Verification items for this drawing (mm, ordinates from the low corner). Coordinates: 2 decimals unless noted, no trailing zeros. Order: outer loops, then holes, each group sorted by start corner. A loop starts at its lowest first (then second) coordinate and runs counter-clockwise, first axis right, second up. Notation, with made-up numbers: (-11, 76.5) - (22, 76.5) arc R30 cw to (22, 106.5) - close; hole circle Ø4 at (34.25, -16.5). An arc over 180 degrees is marked (long way). Use CSV: the item, a comma, the result in double quotes. Start each with the question number.
1) Depth check by flat-ended pin: P1, Ø7.5, axis at x = 17.78, y = 17.78, coming from the +Z side. Enter the tip coordinate at first touch or a pass-through.
2) Sectioned sample at B-B, the plane x = 287.02. Record the cut outline in (y, z).
3) Sectioned sample at A-A, the plane y = 134.62. Record the cut outline in (x, z).
4) Thickness scan on probe 1 along Y at (x, z) = (287.02, 8); probe 2 along Y at (x, z) = (284.5, 10). Record the ranges inside material, lowest first. Write a range as [from, to].
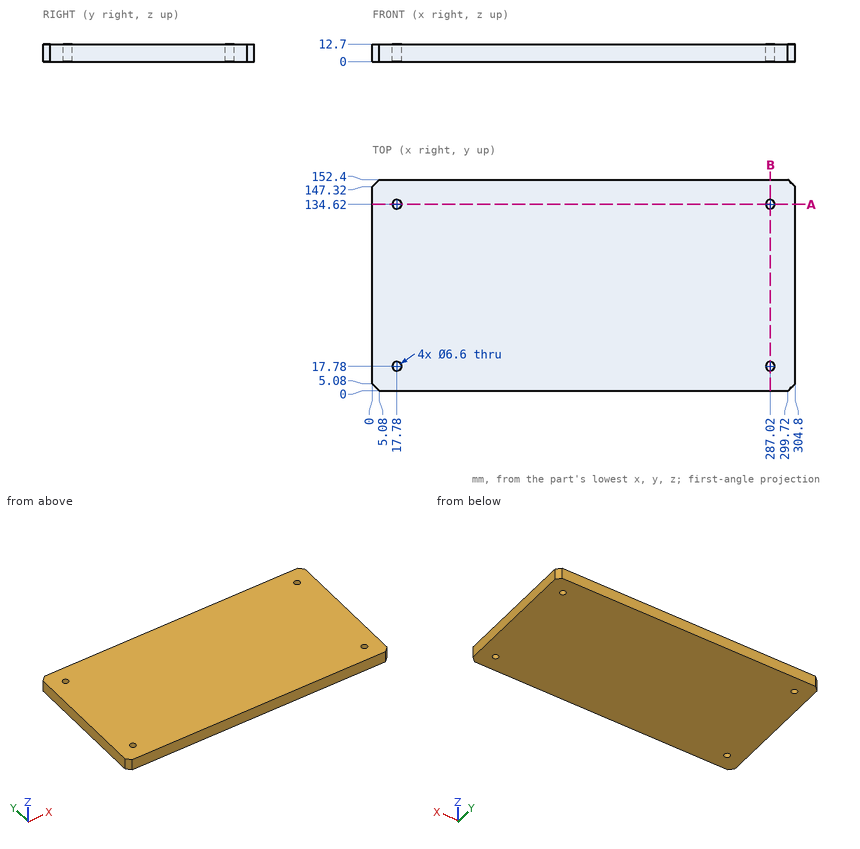
Evaluation:
1,P1,"z = 12.7"
2,outline,"(0, 0) - (14.48, 0) - (14.48, 12.7) - (0, 12.7) - close; (21.08, 0) - (131.32, 0) - (131.32, 12.7) - (21.08, 12.7) - close; (137.92, 0) - (152.4, 0) - (152.4, 12.7) - (137.92, 12.7) - close"
3,outline,"(0, 0) - (14.48, 0) - (14.48, 12.7) - (0, 12.7) - close; (21.08, 0) - (283.72, 0) - (283.72, 12.7) - (21.08, 12.7) - close; (290.32, 0) - (304.8, 0) - (304.8, 12.7) - (290.32, 12.7) - close"
4,probe 1,"[0, 14.48], [21.08, 131.32], [137.92, 152.4]"
4,probe 2,"[0, 15.65], [19.91, 132.49], [136.75, 152.4]"
